The model under review builds one solid part; all positions refer to its coordinate system, in mm. A direction names the side the tool comes from. Give positions to 0.01 mm unless a question says otherwise; leave off trailing zeros. Order: outer loops, then holes, each group sorted by start corner. A loop starts at its lowest first (then second) coordinate and runs counter-clockwise, first axis right, second up. Notation, with made-up numbers: M 44.25,65 L 54.25,65 A23 ccw 54.25,103 Z; hole C 16.25,33.5 d7. An arc over 180 degrees is marked long. One line per question, with ' | ' between items. Start each with the question number.
1. Wall thickness on L1, parallel to Z at x = 2.1, y = 12.7; L2, parallel to Z at x = 0.55, y = 11.5; L3, parallel to Y at x = 0.5, z = 59: over which ranges is each line inside the solid? List them lowest first.
2. Insertion check: P1, Ø4, axis at y = 65.56, z = 23.89, coming from the +X side; P2, Ø1.6, axis at x = 1.5, z = 55.5, coming from the +Y side. Each pin has a flat end and moves straight along its axis. Give the tip position at first contact, or say it passes through.
3. For faces 5 (the face through (2, 0, 39)), 6 (the face through (2, 25.4, 59)), list the 3-axis set-ups (+Z, -Z, +X, -X, +Y, -Y) from which the entire face can be reached by the end or side of a thin tool; tool diameter is ignored.
4. We need section C-C on x = 2.05. Write out the cut boundary in (y, z), then the cut area to 3 significant figures.
5. The part is to be moulded in two halves that separate along Y. For faces 1 (the face through (0, 40, 22)), 2 (the face through (1.57, 41.08, 13.48)), 3 (the face through (1.565, 68.99, 11.646)), 4 (the face through (1.565, 13.878, 65.765)), say which applies: +Y half, -Y half, draft (parallel to the pull), parting line (faces both ways), or undercut.
6. We need section B-B on y = 12.7. Write out the cut boundary in (x, z) (3 decimals), then the cut area to 3 significant figures.
7. We need section A-A on z = 63.5. Write out the cut boundary in (x, y) (3 decimals), then the cut area to 3 significant figures.
8. We need section D-D on z = 38.1. Write out the cut boundary in (x, y) (3 decimals), then the cut area to 3 significant figures.
Autodesk Inventor part; units mm, degrees
ref_plane "YZ Plane" through (0, 0, 0) normal (1, 0, 0) x (0, 1, 0)
ref_plane "XZ Plane" through (0, 0, 0) normal (0, 1, 0) x (-1, 0, 0)
ref_plane "XY Plane" through (0, 0, 0) normal (0, 0, 1) x (1, 0, 0)
sketch "Sketch1" plane through (0, 0, 0) normal (1, 0, 0) x (0, 1, 0)
  line L0 (0, 0) -> (25.4, 0)
  line L1 (25.4, 0) -> (25.4, 76.2)
  line L2 (25.4, 76.2) -> (0, 76.2)
  line L3 (0, 76.2) -> (0, 0)
  line L4 (25.4, 0) -> (33.274, 0)
  line L5 (33.274, 0) -> (105.7201, 23.622)
  line L6 (105.7201, 23.622) -> (97.8461, 47.7707)
  line L7 (97.8461, 47.7707) -> (25.4, 24.1487)
  circle A0 centre (41.4114, 16.0114) radius 2.5527
  circle A1 centre (12.7, 12.7) radius 2.5527
  line L8 (25.4, 24.1487) -> (33.274, 0)
  circle A2 centre (12.7, 38.1) radius 2.5527
  circle A3 centre (12.7, 63.5) radius 2.5527
  circle A4 centre (65.5601, 23.8854) radius 2.5527
  circle A5 centre (89.7088, 31.7594) radius 2.5527
  point P0 (12.7, 0)
  dimension "d0" = 25.4
  dimension "d1" = 76.2
  dimension "d2" = 7.874
  dimension "d3" = 76.2
  dimension "d4" = 25.4
  dimension "d5" = 5.1054
  dimension "d6" = 5.1054
  dimension "d7" = 12.7
  dimension "d8" = 12.7
  dimension "d9" = 12.7
  dimension "d10" = 12.7
  dimension "d20" = 25.4
  dimension "d27" = 25.4
extrude "Extrusion1" add sketch "Sketch1" along normal blind 3.175
fillet "Fillet1" radius 12.7 1 edges at (1.5875, 25.4, 24.1487)
properties part number "Bot_ang_gus"
Entries:
1) L1: z = 0 to 10.15, 15.25 to 35.55, 40.65 to 60.95, 66.05 to 76.2 | L2: z = 0 to 10.45, 14.95 to 35.85, 40.35 to 61.25, 65.75 to 76.2 | L3: y = 0 to 25.4
2) P1: passes through | P2: stops at y = 25.4
3) face 5: +Z, -Z, +X, -X, -Y | face 6: +Z, +X, -X
4) outline: M 0,0 L 33.27,0 L 105.72,23.62 L 97.85,47.77 L 42.04,29.57 A12.7 cw 25.4,41.65 L 25.4,76.2 L 0,76.2 Z; hole C 12.7,12.7 d5.11; hole C 12.7,38.1 d5.11; hole C 12.7,63.5 d5.11; hole C 41.41,16.01 d5.11; hole C 65.56,23.89 d5.11; hole C 89.71,31.76 d5.11 | area: 3,910 mm^2
5) face 1: draft | face 2: undercut | face 3: +Y half | face 4: undercut
6) outline: M 0,0 L 3.175,0 L 3.175,10.147 L 0,10.147 Z; M 0,15.253 L 3.175,15.253 L 3.175,35.547 L 0,35.547 Z; M 0,40.653 L 3.175,40.653 L 3.175,60.947 L 0,60.947 Z; M 0,66.053 L 3.175,66.053 L 3.175,76.2 L 0,76.2 Z | area: 193 mm^2
7) outline: M 0,0 L 3.175,0 L 3.175,10.147 L 0,10.147 Z; M 0,15.253 L 3.175,15.253 L 3.175,25.4 L 0,25.4 Z | area: 64.4 mm^2
8) outline: M 0,0 L 3.175,0 L 3.175,10.147 L 0,10.147 Z; M 0,15.253 L 3.175,15.253 L 3.175,25.906 L 0,25.906 Z; M 0,68.187 L 3.175,68.187 L 3.175,100.999 L 0,100.999 Z | area: 170 mm^2
